Part model, mm, in its own coordinate system. A direction names the side the tool comes from. Give positions to 0.01 mm unless a question says otherwise; leave off trailing zeros. Write each loop counter-clockwise with the first axis right and the second up, starting at its lowest first coordinate (ties: lowest second). Pieces come first, ordered by that corner, then holes.
from build123d import *

# Parameters (mm, degrees)
PAD001_DEPTH        = 2
SKETCH008_R         = 1
POCKET006_DEPTH     = 5
SKETCH010_R         = 2.07
POCKET007_DEPTH     = 2
FILLET002_R         = 0.4
FILLET002_FACE5_R   = 2.07
FILLET002_FACE5_R_2 = 1
POCKET011_DEPTH     = 0.1


with BuildPart() as part:
    # Sketch007 → Pad001 (new body)
    with BuildSketch(Plane.XY):
        with BuildLine():
            ThreePointArc((6.0419601085, -0.5), (12, 0), (6.0419601085, 0.5))
            Line((1.99959996, 0.5), (6.0419601085, 0.5))
            Line((1.99959996, 2.84), (1.99959996, 0.5))
            ThreePointArc((1.99959996, 2.84), (0, 4.8), (-1.99959996, 2.84))
            Line((-1.99959996, 2.84), (-1.99959996, 0.5))
            Line((-6.0419601085, 0.5), (-1.99959996, 0.5))
            ThreePointArc((-6.0419601085, 0.5), (-12, 0), (-6.0419601085, -0.5))
            Line((-6.0419601085, -0.5), (-3, -0.5))
            Line((-3, -0.5), (-3, -2))
            Line((-3, -2), (-2, -2))
            Line((-2, -2), (-2, -0.5))
            Line((-2, -0.5), (2, -0.5))
            Line((2, -0.5), (2, -2))
            Line((2, -2), (3, -2))
            Line((3, -2), (3, -0.5))
            Line((3, -0.5), (6.0419601085, -0.5))
        make_face()
    extrude(amount=PAD001_DEPTH)

    # Sketch008 (on Face18 of Pad001) → Pocket006 (cut)
    with BuildSketch(Plane.XY.offset(2)):
        with Locations((0, 2.88)):
            Circle(SKETCH008_R)
    extrude(amount=-POCKET006_DEPTH, mode=Mode.SUBTRACT)

    # Sketch010 (on Face5 of Pocket006) → Pocket007 (cut)
    with BuildSketch(Plane.XY.offset(2)):
        with Locations((-9.06, 0)):
            Circle(SKETCH010_R)
        with Locations((9.06, 0)):
            Circle(SKETCH010_R)
    extrude(amount=-POCKET007_DEPTH, mode=Mode.SUBTRACT)

    # Fillet002
    fillet002_edges = [part.edges().sort_by_distance(p)[0] for p in [
        (-3, -2, 1),
        (-2, -2, 1),
        (-3, -0.5, 1),
        (-2, -0.5, 1),
        (2, -0.5, 1),
        (2, -2, 1),
        (3, -2, 1),
        (3, -0.5, 1),
    ]]
    fillet(fillet002_edges, radius=FILLET002_R)

    # Fillet002 Face5 → Pocket011 (cut)
    with BuildSketch(Plane(origin=(0, 0.4471888212, 2), x_dir=(0, 1, 0), z_dir=(0, 0, 1))):
        with BuildLine():
            Line((-0.9471888212, 6.0419601085), (-0.9471888212, 3.4))
            ThreePointArc((-0.9471888212, 3.4), (-1.0643461087, 3.1171572875), (-1.3471888212, 3))
            Line((-1.3471888212, 3), (-2.0471888212, 3))
            ThreePointArc((-2.0471888212, 3), (-2.3300315337, 2.8828427125), (-2.4471888212, 2.6))
            Line((-2.4471888212, 2.6), (-2.4471888212, 2.4))
            ThreePointArc((-2.4471888212, 2.4), (-2.3300315337, 2.1171572875), (-2.0471888212, 2))
            Line((-2.0471888212, 2), (-1.3471888212, 2))
            ThreePointArc((-1.3471888212, 2), (-1.0643461087, 1.8828427125), (-0.9471888212, 1.6))
            Line((-0.9471888212, 1.6), (-0.9471888212, -1.6))
            ThreePointArc((-0.9471888212, -1.6), (-1.0643461087, -1.8828427125), (-1.3471888212, -2))
            Line((-1.3471888212, -2), (-2.0471888212, -2))
            ThreePointArc((-2.0471888212, -2), (-2.3300315337, -2.1171572875), (-2.4471888212, -2.4))
            Line((-2.4471888212, -2.4), (-2.4471888212, -2.6))
            ThreePointArc((-2.4471888212, -2.6), (-2.3300315337, -2.8828427125), (-2.0471888212, -3))
            Line((-2.0471888212, -3), (-1.3471888212, -3))
            ThreePointArc((-1.3471888212, -3), (-1.0643461087, -3.1171572875), (-0.9471888212, -3.4))
            Line((-0.9471888212, -3.4), (-0.9471888212, -6.0419601085))
            ThreePointArc((-0.9471888212, -6.0419601085), (-0.4471888212, -12), (0.0528111788, -6.0419601085))
            Line((0.0528111788, -6.0419601085), (0.0528111788, -1.99959996))
            Line((0.0528111788, -1.99959996), (2.3928111788, -1.99959996))
            ThreePointArc((2.3928111788, -1.99959996), (4.3528111788, 0), (2.3928111788, 1.99959996))
            Line((2.3928111788, 1.99959996), (0.0528111788, 1.99959996))
            Line((0.0528111788, 1.99959996), (0.0528111788, 6.0419601085))
            ThreePointArc((0.0528111788, 6.0419601085), (-0.4471888212, 12), (-0.9471888212, 6.0419601085))
        make_face()
        with Locations((-0.4471888212, 9.06)):
            Circle(FILLET002_FACE5_R, mode=Mode.SUBTRACT)
        with Locations((-0.4471888212, -9.06)):
            Circle(FILLET002_FACE5_R, mode=Mode.SUBTRACT)
        with Locations((2.4328111788, 0)):
            Circle(FILLET002_FACE5_R_2, mode=Mode.SUBTRACT)
    extrude(amount=-POCKET011_DEPTH, mode=Mode.SUBTRACT)


with BuildPart() as part_1:
    # Body001 placement: moved
    add(part.part.moved(Location((0, 0, 3))))


solid = part_1.part
1) 3-axis set-ups, long thin cutter, end or side, ignore diameter. For faces 4 (the flat face through (4, 0.5, 4)), 5 (the cylindrical face through (-0.2, 1.9, 4)), 6 (the flat face through (-5, -0.5, 4)): which of +Z, -Z, +X, -X, +Y, -Y reach the whole face in a straight line?
Check result:
face 4: +Z, -Z, +Y
face 5: +Z, -Z
face 6: +Z, -Z, -Y
2) Saw through at D-D (z = 3.7). Write the cut outline in (x, y).
Check result:
outline: (-6.04, -0.5) - (-3.4, -0.5) arc R0.4 cw to (-3, -0.9) - (-3, -1.6) arc R0.4 ccw to (-2.6, -2) - (-2.4, -2) arc R0.4 ccw to (-2, -1.6) - (-2, -0.9) arc R0.4 cw to (-1.6, -0.5) - (1.6, -0.5) arc R0.4 cw to (2, -0.9) - (2, -1.6) arc R0.4 ccw to (2.4, -2) - (2.6, -2) arc R0.4 ccw to (3, -1.6) - (3, -0.9) arc R0.4 cw to (3.4, -0.5) - (6.04, -0.5) arc R3 ccw (long way) to (6.04, 0.5) - (2, 0.5) - (2, 2.84) arc R2 ccw to (-2, 2.84) - (-2, 0.5) - (-6.04, 0.5) arc R3 ccw (long way) to start; hole circle Ø4.14 at (-9.06, 0); hole circle Ø2 at (0, 2.88); hole circle Ø4.14 at (9.06, 0)
3) Mould opens along X. For faces 1 (the cylindrical face through (12, 0, 4)), 2 (the flat face through (0, 0, 4.9)), 3 (the flat face through (5, -0.5, 4)) say: +X half, -X half, draft (parallel to the pull), parting line (faces both ways), or undercut.
Check result:
face 1: undercut
face 2: draft
face 3: undercut
4) Saw through at B-B (x = 0). Write the cut outline in (y, z).
Check result:
outline: (-0.5, 3) - (1.88, 3) - (1.88, 4.9) - (-0.5, 4.9) - close; (3.88, 3) - (4.8, 3) - (4.8, 4.9) - (3.88, 4.9) - close
5) Drill centre lines: L1, parallel to Y at x = 9.06, z = 4.5; L2, parallel to X at y = 2.5, z = 3.55; L3, parallel to X at y = -1.5, z = 4.6. Where is each one in solid material? Low to high.
Check result:
L1: y = -3 to -2.07, 2.07 to 3
L2: x = -10.66 to -7.34, -2 to -0.92, 0.92 to 2, 7.34 to 10.66
L3: x = -11.6 to -10.49, -7.63 to -6.4, -3 to -2, 2 to 3, 6.4 to 7.63, 10.49 to 11.6
6) Saw through at C-C (y = 3.25). Write the cut outline in (x, z), and give its area (3 significant figures).
Check result:
outline: (-1.95, 3) - (-0.93, 3) - (-0.93, 4.9) - (-1.95, 4.9) - close; (0.93, 3) - (1.95, 3) - (1.95, 4.9) - (0.93, 4.9) - close
area: 3.87 mm2
7) Saw through at A-A (y = 0). Write the cut outline in (x, z).
Check result:
outline: (-12, 3) - (-11.13, 3) - (-11.13, 4.9) - (-12, 4.9) - close; (-6.99, 3) - (6.99, 3) - (6.99, 4.9) - (-6.99, 4.9) - close; (11.13, 3) - (12, 3) - (12, 4.9) - (11.13, 4.9) - close
8) Flat gauge pins, fed straight in: P1, Ø0.6, axis at x = 5, z = 3.5, coming from the +Y side; P2, Ø0.6, axis at y = 2, z = 4, coming from the +X side; P3, Ø3.5, axis at x = -9.06, y = 0, coming from the +Z side; P4, Ø1, axis at x = -5.5, z = 4, coming from the -Y side. Where does each tip first touch, or does it go through?
Check result:
P1: stops at y = 0.5
P2: stops at x = 11.47
P3: passes through
P4: stops at y = -0.5
